from build123d import *

# Parameters (mm, degrees)
EXTRUDE003_DEPTH = 1.5
ARRAY001_COUNT   = 12
SKETCH017_R      = 47.5
SKETCH017_R_2    = 42.5
EXTRUDE002_DEPTH = 2
SKETCH021_R      = 10
EXTRUDE004_DEPTH = 2.5
TUBE001_R        = 100
TUBE001_R_2      = 4
TUBE001_DEPTH    = 6


with BuildPart() as tenminutemarksarray:
    # Sketch014 → Extrude003 (new body)
    with BuildSketch(Plane.XY):
        with BuildLine():
            Line((-1.5, 84.986764), (-1.5, 92.487837))
            ThreePointArc((1.5, 92.487837), (0, 92.5), (-1.5, 92.487837))
            Line((1.5, 84.986764), (1.5, 92.487837))
            ThreePointArc((1.5, 84.986764), (0, 85), (-1.5, 84.986764))
        make_face()
    extrude(amount=-EXTRUDE003_DEPTH)

    # Array001: TenMinuteMarksArray ×12 about axis
    array001_axis = Axis((0, 0, 0), (0, 0, 1))


with BuildPart() as tenminutemarksarray_1:
    add(tenminutemarksarray.part)
    for i in range(1, ARRAY001_COUNT):
        add(tenminutemarksarray.part.rotate(array001_axis, i * 360 / ARRAY001_COUNT))


with BuildPart() as obj1:
    # Sketch017 → Extrude002 (new body)
    with BuildSketch(Plane.XY):
        Circle(SKETCH017_R)
        Circle(SKETCH017_R_2, mode=Mode.SUBTRACT)
    extrude(amount=-EXTRUDE002_DEPTH)


with BuildPart() as dialplatecutouts:
    # Sketch021 → Extrude004 (new body)
    with BuildSketch(Plane.XY.offset(-3.5)):
        with Locations((0, 35)):
            Circle(SKETCH021_R)
        with Locations((0, -35)):
            Circle(SKETCH021_R)
    extrude(amount=-EXTRUDE004_DEPTH)

    # Fusion: union TenMinuteMarksArray, obj1
    add(tenminutemarksarray_1.part)
    add(obj1.part)


with BuildPart() as dialplate:
    # Tube001 → Tube001 (new body)
    with BuildSketch(Plane.XY.offset(-6)):
        Circle(TUBE001_R)
        Circle(TUBE001_R_2, mode=Mode.SUBTRACT)
    extrude(amount=TUBE001_DEPTH)

    # Cut: cut DialPlateCutouts
    add(dialplatecutouts.part, mode=Mode.SUBTRACT)


solid = dialplate.part
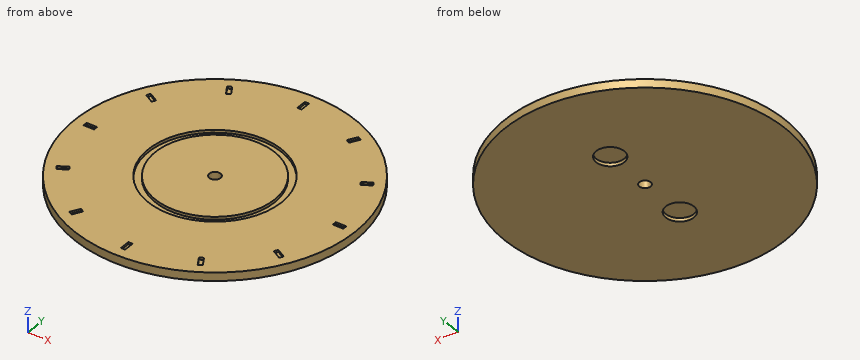
The model under review builds one solid part; all positions refer to its coordinate system, in mm. Round coordinates to 2 decimals unless told otherwise and drop trailing zeros. Write each loop counter-clockwise with the first axis right and the second up, starting at its lowest first coordinate (ties: lowest second). Pieces come first, ordered by that corner, then holes. Notation, with made-up numbers: M 58,-33.75 L 101,-33.75 A31 ccw 101,0.25 Z; hole C -7,63.25 d4. An arc over 180 degrees is marked long. Use a Markdown table: item, result. Add a question column.
Q1. We need section D-D, the plane y = -8.5. State the section outline as (x, z) points.
Q2. We need section C-C, the plane y = 35. State the section outline as (x, z) points, plus the area to 3 significant figures.
Q3. We need section B-B, the plane z = -4.55. State the section outline as (x, y) points.
Q4. We need section A-A, the plane x = -26. State the section outline as (y, z) points.
Q5. To check wall thickness, follow line 1 (Y direction, x = 0, z = -1.3); line 2 (Y direction, x = 0, z = -4.5); line 3 (Y direction, x = -33.5, z = -0.25). State the ranges of each line that lie inside material, in increasing order.
Q6. Insertion check: pin 1 (1.6 mm diameter, centred on x = 90, z = -1, fed in from -Y); pin 2 (1.2 mm diameter, centred on y = 88, z = -1, fed in from -X); pin 3 (1.6 mm diameter, centred on x = 89, z = -0.5, fed in from +Y). Each pin has a flat end and moves straight along its axis. Give the tip position at first contact, or say it passes through.
Findings below:
| question | item | result |
|---|---|---|
| 1 | outline | M -99.64,-6 L 99.64,-6 L 99.64,0 L 46.73,0 L 46.73,-2 L 41.64,-2 L 41.64,0 L -41.64,0 L -41.64,-2 L -46.73,-2 L -46.73,0 L -99.64,0 Z |
| 2 | outline | M -93.67,-6 L -10,-6 L -10,-3.5 L 10,-3.5 L 10,-6 L 93.67,-6 L 93.67,0 L 32.11,0 L 32.11,-2 L 24.11,-2 L 24.11,0 L -24.11,0 L -24.11,-2 L -32.11,-2 L -32.11,0 L -93.67,0 Z |
| 2 | area | 1,040 mm² |
| 3 | outline | C 0,0 d200; hole C 0,-35 d20; hole C 0,35 d20; hole C 0,0 d8 |
| 4 | outline | M -96.56,-6 L 96.56,-6 L 96.56,0 L 39.75,0 L 39.75,-2 L 33.62,-2 L 33.62,0 L -33.62,0 L -33.62,-2 L -39.75,-2 L -39.75,0 L -96.56,0 Z |
| 5 | line 1 | y = -100 to -92.5, -85 to -47.5, -42.5 to -4, 4 to 42.5, 47.5 to 85, 92.5 to 100 |
| 5 | line 2 | y = -100 to -45, -25 to -4, 4 to 25, 45 to 100 |
| 5 | line 3 | y = -94.22 to -33.67, -26.15 to 26.15, 33.67 to 94.22 |
| 6 | pin 1 | stops at y = -45.2 |
| 6 | pin 2 | stops at x = -48.59 |
| 6 | pin 3 | stops at y = 47.12 |
